Could you check a few things on this model? Use its own coordinates, in mm. A direction names the side the tool comes from. Coordinates: 2 decimals unless noted, no trailing zeros. Order: outer loops, then holes, each group sorted by start corner. A loop starts at its lowest first (then second) coordinate and runs counter-clockwise, first axis right, second up. Notation, with made-up numbers: (-13.5, 45.25) - (9.5, 45.25) arc R28 cw to (9.5, 64.25) - close; hole circle Ø9 at (-31.75, 42). An arc over 180 degrees is marked (long way). One line per item, written item: value.
from build123d import *

# Parameters (mm, degrees)
SKETCH_1_R          = 2.5
EXTRUDE_1_DEPTH     = 121
SKETCH_2_R          = 4.5
EXTRUDE_2_DEPTH     = 3
SKETCH_4_W          = 1.5
SKETCH_4_H          = 10.936891942
CUT_EXTRUDE_1_DEPTH = 2


with BuildPart() as part:
    # 草图1 → 凸台-拉伸1 (new body)
    with BuildSketch(Plane.XY):
        Circle(SKETCH_1_R)
    extrude(amount=EXTRUDE_1_DEPTH)

    # 草图2 → 凸台-拉伸2 (add)
    with BuildSketch(Plane.XY.offset(121)):
        Circle(SKETCH_2_R)
    extrude(amount=EXTRUDE_2_DEPTH)

    # 草图4 → 切除-拉伸1 (cut)
    with BuildSketch(Plane.XY.offset(124)):
        Rectangle(SKETCH_4_W, SKETCH_4_H)
    extrude(amount=-CUT_EXTRUDE_1_DEPTH, mode=Mode.SUBTRACT)


solid = part.part
Item 1: I'm going to push flat-ended pins straight in: pin 1 Ø5 at (y, z) = (1, 30.5) entering from +X; pin 2 Ø1 at (x, z) = (1, 96) entering from -Y; pin 3 Ø2 at (y, z) = (1.5, 123) entering from -X. Where does each tip first touch, or does it pass through?
Conclusion:
pin 1: x = 2.5
pin 2: y = -2.45
pin 3: x = -4.47
Item 2: If I drill on probe 1 along Z at (x, y) = (-1.25, 3.5); probe 2 along Z at (x, y) = (-0.25, -3.25); probe 3 along X at (y, z) = (-0.25, 83.5), over which ranges is the centre line in solid material (lowest first)?
Conclusion:
probe 1: 121 to 124
probe 2: 121 to 122
probe 3: -2.49 to 2.49
Item 3: I want a section at B-B on z = 104.5. Please give me the cut outline in (x, y).
Conclusion:
outline: circle Ø5 at (0, 0)
Item 4: For faces 1 (the face through (-2, 0, 124)), 2 (the face through (2, -2, 121)), which set-ups out of +Z, -Z, +X, -X, +Y, -Y let a thin tool reach every point of the face, with its end or its side?
Conclusion:
face 1: +Z, +X, -X, +Y, -Y
face 2: -Z
Item 5: I want a section at A-A on y = 0. Please give me the cut outline in (x, z), then the cut area to 3 significant figures.
Conclusion:
outline: (-4.5, 121) - (-2.5, 121) - (-2.5, 0) - (2.5, 0) - (2.5, 121) - (4.5, 121) - (4.5, 124) - (0.75, 124) - (0.75, 122) - (-0.75, 122) - (-0.75, 124) - (-4.5, 124) - close
area: 629 mm²
Item 6: Thinking about a two-plate mould opening in X: for faces 3 (the face through (-0.75, 0, 123)), 4 (the face through (2, 0, 124)), 5 (the face through (-0.54, -2.44, 59.65)), 6 (the face through (0.75, 0, 123)), which applies, pulls with the +X half, pulls with the -X half, needs draft (parallel to the pull), parting line crosses it, or undercut?
Conclusion:
face 3: undercut
face 4: needs draft
face 5: parting line crosses it
face 6: undercut
